from build123d import *

# Parameters (mm, degrees)
SKETCH_1_R          = 17.5
SKETCH_1_R_2        = 10
SKETCH_1_R_3        = 1.5
SKETCH_1_R_4        = 4
EXTRUDE_1_DEPTH     = 23
SKETCH_1_4_R        = 17.5
SKETCH_1_4_R_2      = 10
CUT_EXTRUDE_1_DEPTH = 20
EXTRUDE_START       = -3
SKETCH_1_5_R        = 17.5
SKETCH_1_5_R_2      = 10
SKETCH_1_5_R_3      = 1.5
SKETCH_1_5_R_4      = 4
EXTRUDE_3_DEPTH     = 3
SKETCH_3_R          = 1
CUT_EXTRUDE_2_DEPTH = 9


with BuildPart() as part:
    # Sketch 1 → Extrude 1 (new body)
    # profile 1 of 2: a face of its own
    with BuildSketch(Plane.XY):
        Circle(SKETCH_1_R)
        Circle(SKETCH_1_R_2, mode=Mode.SUBTRACT)
    # profile 2 of 2: a face of its own
    with BuildSketch(Plane.XY):
        Circle(SKETCH_1_R_2)
        with Locations((0, 7)):
            Circle(SKETCH_1_R_3, mode=Mode.SUBTRACT)
        with Locations((7, 0)):
            Circle(SKETCH_1_R_3, mode=Mode.SUBTRACT)
        with Locations((0, -7)):
            Circle(SKETCH_1_R_3, mode=Mode.SUBTRACT)
        with Locations((-7, 0)):
            Circle(SKETCH_1_R_3, mode=Mode.SUBTRACT)
        Circle(SKETCH_1_R_4, mode=Mode.SUBTRACT)
    extrude(amount=EXTRUDE_1_DEPTH)

    # Sketch 1_4 → Cut-Extrude 1 (cut)
    with BuildSketch(Plane.XY):
        Circle(SKETCH_1_4_R)
        Circle(SKETCH_1_4_R_2, mode=Mode.SUBTRACT)
    extrude(amount=CUT_EXTRUDE_1_DEPTH, mode=Mode.SUBTRACT)

    # Sketch 1_5 → Extrude 3 (add)
    # profile 1 of 2: a face of its own
    with BuildSketch(Plane.XY.offset(EXTRUDE_START)):
        Circle(SKETCH_1_5_R)
        Circle(SKETCH_1_5_R_2, mode=Mode.SUBTRACT)
    # profile 2 of 2: a face of its own
    with BuildSketch(Plane.XY.offset(EXTRUDE_START)):
        Circle(SKETCH_1_5_R_2)
        with Locations((0, 7)):
            Circle(SKETCH_1_5_R_3, mode=Mode.SUBTRACT)
        with Locations((7, 0)):
            Circle(SKETCH_1_5_R_3, mode=Mode.SUBTRACT)
        with Locations((0, -7)):
            Circle(SKETCH_1_5_R_3, mode=Mode.SUBTRACT)
        with Locations((-7, 0)):
            Circle(SKETCH_1_5_R_3, mode=Mode.SUBTRACT)
        Circle(SKETCH_1_5_R_4, mode=Mode.SUBTRACT)
    extrude(amount=EXTRUDE_3_DEPTH)

    # Sketch 3 → Cut-Extrude 2 (cut)
    with BuildSketch(Plane(origin=(7.071067812, 7.071067812, 0), x_dir=(0.7071067811865488, -0.7071067811865462, 0), z_dir=(0.7071067811865462, 0.7071067811865488, 0))):
        with Locations(Location((0, -10, 0), (0, 0, 180))):
            Circle(SKETCH_3_R)
    extrude(amount=-CUT_EXTRUDE_2_DEPTH, mode=Mode.SUBTRACT)


solid = part.part
The listing builds one solid part. Answer for the finished solid, in the listing's coordinates (mm). A direction names the side the tool comes from. Give positions to 0.01 mm unless a question says otherwise; leave off trailing zeros. Write each loop counter-clockwise with the first axis right and the second up, starting at its lowest first coordinate (ties: lowest second). Pieces come first, ordered by that corner, then holes.
1) Given P1, Ø5, axis at x = 0, y = 7, coming from the +Z side; P2, Ø3, axis at y = 9, z = 7.5, coming from the +X side; P3, Ø1.5, axis at y = -8, z = 3.5, coming from the -X side; P4, Ø12, axis at x = -1.5, z = 10, coming from the -Y side, each flat-ended and moving along its own axis, determine where each tip first touches the part or whether it passes through.
2) Section A-A (y = 0) is taken. Write down the section's boundary in (x, z), and give its area (3 significant figures).
3) Find the intervals of material crossed by L1, parallel to Y at x = 0, z = 10; L2, parallel to Z at x = -8, y = 14.5; L3, parallel to Y at x = 1, z = 14.5, in increasing order.
4) A tool of negligible diameter and unlimited length cuts with its end or side. For faces 4 (the face through (8, -8, 0)), 5 (the face through (5.5, 0.07, 9.82)), from which of +Z, -Z, +X, -X, +Y, -Y can it reach the whole face along a straight path? Write none if from no direction.
5) For a pull along Z with two mould halves and no side action, classify faces 1 (the face through (-0.325, -8.464, 9.818)), 2 (the face through (-2.17, -9.76, 9.86)), 3 (the face through (4, -4, 23)) as pulls with the +Z half, pulls with the -Z half, needs draft (parallel to the pull), parting line crosses it, or undercut.
6) Section C-C (x = -14) is taken. Write down the section's boundary in (y, z).
7) Section D-D (y = -13) is taken. Write down the section's boundary in (x, z).
Response:
1. P1: stops at z = 23
1. P2: stops at x = 6.61
1. P3: stops at x = -6.89
1. P4: stops at y = -10
2. outline: (-17.5, -3) - (-8.5, -3) - (-8.5, 23) - (-17.5, 23) - (-17.5, 20) - (-10, 20) - (-10, 0) - (-17.5, 0) - close; (-5.5, -3) - (-4, -3) - (-4, 23) - (-5.5, 23) - close; (4, -3) - (5.5, -3) - (5.5, 23) - (4, 23) - close; (8.5, -3) - (17.5, -3) - (17.5, 0) - (10, 0) - (10, 20) - (17.5, 20) - (17.5, 23) - (8.5, 23) - close
2. area: 246 mm2
3. L1: y = -10 to -8.5, -5.5 to -4, 4 to 5.5, 8.5 to 10
3. L2: z = -3 to 0, 20 to 23
3. L3: y = -9.95 to -8.12, -5.88 to -3.87, 3.87 to 5.88, 8.12 to 9.95
4. face 4: none
4. face 5: +Z, -Z
5. face 1: needs draft
5. face 2: undercut
5. face 3: pulls with the +Z half
6. outline: (-10.5, -3) - (10.5, -3) - (10.5, 0) - (-10.5, 0) - close; (-10.5, 20) - (10.5, 20) - (10.5, 23) - (-10.5, 23) - close
7. outline: (-11.72, -3) - (11.72, -3) - (11.72, 0) - (-11.72, 0) - close; (-11.72, 20) - (11.72, 20) - (11.72, 23) - (-11.72, 23) - close
